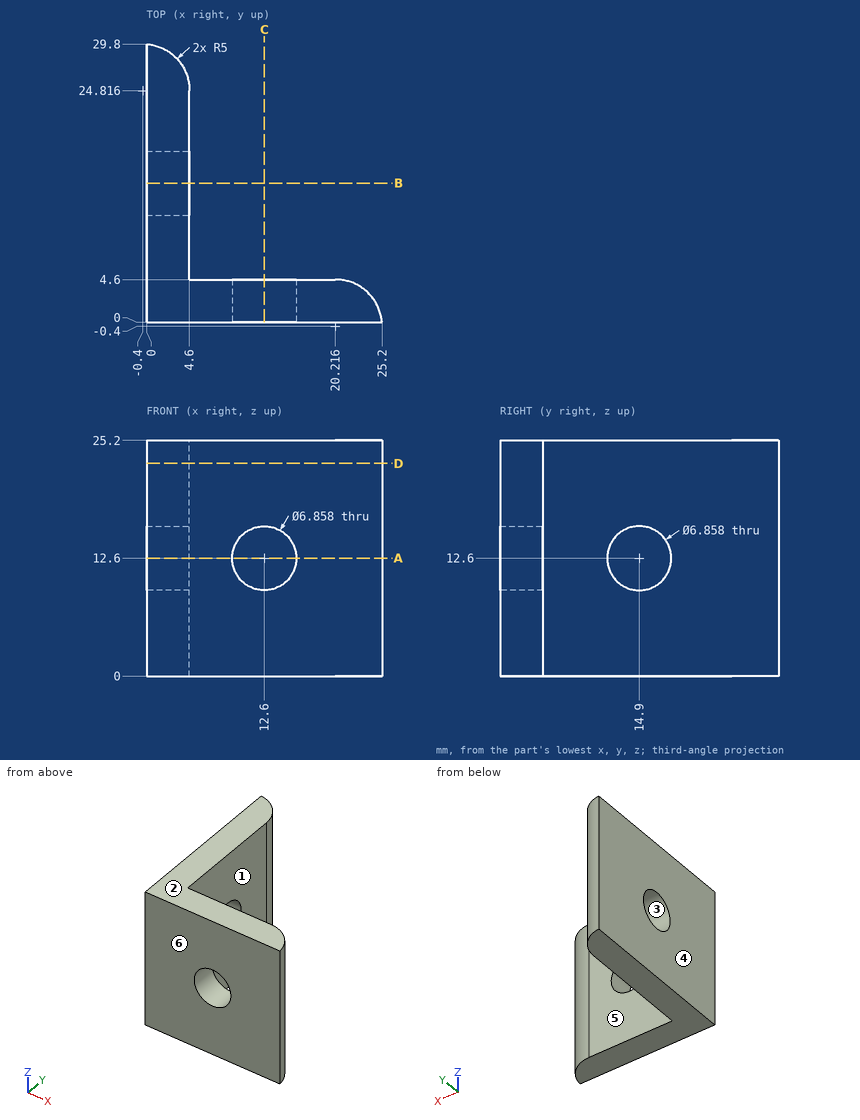
The figure shows three views and two pictorial views of one solid part (mm, origin at its lowest corner). Answer the questions. A direction names the side the tool comes from. Round coordinates to 2 decimals unless told otherwise and drop trailing zeros. Write each loop counter-clockwise with the first axis right and the second up, starting at its lowest first coordinate (ties: lowest second). Pieces come first, ordered by that corner, then holes. Notation, with made-up numbers: (-23, 76) - (27, 76) arc R22 cw to (27, 82) - close; hole circle Ø10 at (62.5, 1). An arc over 180 degrees is marked (long way). Answer in a Markdown table with one row per item. Add a question column.
1. Find the intervals of material crossed by line 1 along Z through (x, y) = (12.25, 1.5); line 2 along Y through (x, z) = (7.5, 6.75), in increasing order. Write a range as from..to.
2. A cutting plane is placed at A-A, the plane z = 12.6. Determine the outline of the cut face in (x, y), and give its area (3 significant figures).
3. Given pin 1 (4 mm diameter, centred on x = 22.5, y = 5, fed in from +Z); pin 2 (5.5 mm diameter, centred on y = 14.9, z = 12.6, fed in from +X); pin 3 (4 mm diameter, centred on y = 13, z = 6.5, fed in from +X); pin 4 (12.5 mm diameter, centred on x = 16, z = 8.5, fed in from +Y), each flat-ended and moving along its own axis, determine where each tip first touches the part or whether it passes through.
4. The mould has two halves that part along Y. Classify the marked faces 3, 4, 5 and 6: +Y half, -Y half, draft (parallel to the pull), parting line (faces both ways), or undercut.
5. A cutting plane is placed at B-B, the plane y = 14.9. Determine the outline of the cut face in (x, z).
6. A cutting plane is placed at D-D, the plane z = 22.75. Determine the outline of the cut face in (x, y).
7. For the marked faces 1 and 2, determine the directions among +Z, -Z, +X, -X, +Y, -Y from which every point of the face is accessible in a straight line to the end or side of a thin tool.
Worked out:
| question | item | result |
|---|---|---|
| 1 | line 1 | 0..9.19, 16.01..25.2 |
| 1 | line 2 | 0..4.6 |
| 2 | outline | (0, 0) - (9.17, 0) - (9.17, 4.6) - (4.6, 4.6) - (4.6, 11.47) - (0, 11.47) - close; (0, 18.33) - (4.6, 18.33) - (4.6, 24.82) arc R5 ccw to (0, 29.8) - close; (16.03, 0) - (25.2, 0) arc R5 ccw to (20.22, 4.6) - (16.03, 4.6) - close |
| 2 | area | 158 mm^2 |
| 3 | pin 1 | z = 25.2 |
| 3 | pin 2 | through |
| 3 | pin 3 | x = 4.6 |
| 3 | pin 4 | y = 4.6 |
| 4 | face 3 | undercut |
| 4 | face 4 | draft |
| 4 | face 5 | +Y half |
| 4 | face 6 | -Y half |
| 5 | outline | (0, 0) - (4.6, 0) - (4.6, 9.17) - (0, 9.17) - close; (0, 16.03) - (4.6, 16.03) - (4.6, 25.2) - (0, 25.2) - close |
| 6 | outline | (0, 0) - (25.2, 0) arc R5 ccw to (20.22, 4.6) - (4.6, 4.6) - (4.6, 24.82) arc R5 ccw to (0, 29.8) - close |
| 7 | face 1 | +Z, -Z, +X, +Y |
| 7 | face 2 | +Z, +X, -X, +Y, -Y |
